The listing builds one solid part. Answer for the finished solid, in the listing's coordinates (mm). Face numbers are marked on the shaded views. Give positions to 0.01 mm unless a question says otherwise; leave off trailing zeros. Loops run counter-clockwise (first coordinate to the right, second up) from the corner with the lowest first, then second, coordinate; pieces in that order, holes last. Notation, with made-up numbers: M 31,52 L 51,52 A15 ccw 51,62 Z; hole C -23.75,27.25 d4. An arc over 180 degrees is marked long. Return JSON: item names as keys, results as strings.
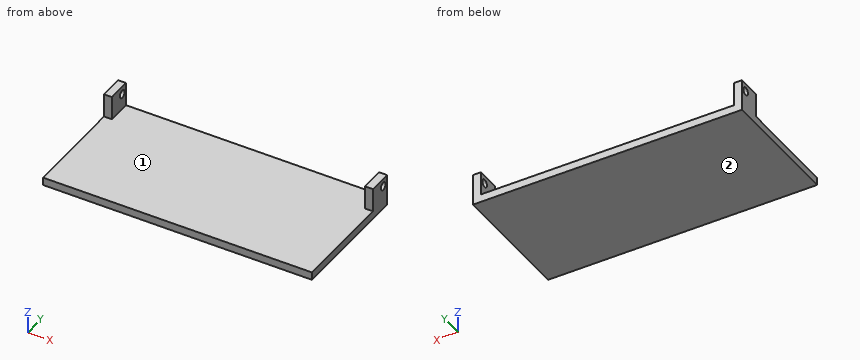
from build123d import *

# Parameters (mm, degrees)
SKETCH_1_W      = 170
SKETCH_1_H      = 80
EXTRUDE_1_DEPTH = 5
SKETCH_2_W      = 20
SKETCH_2_H      = 15
SKETCH_2_R      = 2.5
EXTRUDE_2_DEPTH = 5
EXTRUDE_START   = -5
SKETCH_3_W      = 20
SKETCH_3_H      = 15
SKETCH_3_R      = 2.5
EXTRUDE_3_DEPTH = 5


with BuildPart() as part:
    # 草图1 → 凸台-拉伸1 (new body)
    with BuildSketch(Plane.XY):
        with Locations((-2.943722944, -40)):
            Rectangle(SKETCH_1_W, SKETCH_1_H)
    extrude(amount=EXTRUDE_1_DEPTH)

    # 草图2 → 凸台-拉伸2 (add)
    with BuildSketch(Plane.ZY.offset(87.943722944)):
        with Locations((10, -7.5)):
            Rectangle(SKETCH_2_W, SKETCH_2_H)
        with Locations((15, -4)):
            Circle(SKETCH_2_R, mode=Mode.SUBTRACT)
    extrude(amount=-EXTRUDE_2_DEPTH)

    # 草图3 → 凸台-拉伸3 (add)
    with BuildSketch(Plane(origin=(82.056277056, 0, 0), x_dir=(0, 0, -1), z_dir=(1, 0, 0)).offset(EXTRUDE_START)):
        with Locations((-10, -7.5)):
            Rectangle(SKETCH_3_W, SKETCH_3_H)
        with Locations(Location((-15, -4, 0), (0, 0, 180))):
            Circle(SKETCH_3_R, mode=Mode.SUBTRACT)
    extrude(amount=EXTRUDE_3_DEPTH)


solid = part.part
(1) Straight lines are drawn through the part: line 1 along Y through (x, z) = (-84.1, 15); line 2 along Z through (x, y) = (28, -62); line 3 along X through (y, z) = (-10, 11.25). For each, find the intervals that lie inside material, in ascending order.
Values follow:
{"line 1": "-15 to -6.5, -1.5 to 0", "line 2": "0 to 5", "line 3": "-87.94 to -82.94, 77.06 to 82.06"}
(2) The part is cut by section C-C (x = -18.5). Determine the outline of the cut face in (y, z).
Values follow:
{"outline": "M -80,0 L 0,0 L 0,5 L -80,5 Z"}
(3) Given pin 1 (1.5 mm diameter, centred on x = -84, z = 15.5, fed in from -Y); pin 2 (3 mm diameter, centred on y = -4, z = 15, fed in from -X); pin 3 (4 mm diameter, centred on x = -55, y = -57.5, fed in from +Z), each flat-ended and moving along its own axis, determine where each tip first touches the part or whether it passes through.
Values follow:
{"pin 1": "y = -15", "pin 2": "through", "pin 3": "z = 5"}
(4) The part is cut by section B-B (z = 15). Determine the outline of the cut face in (x, y), and give its area (3 significant figures).
Values follow:
{"outline": "M -87.94,-15 L -82.94,-15 L -82.94,-6.5 L -87.94,-6.5 Z; M -87.94,-1.5 L -82.94,-1.5 L -82.94,0 L -87.94,0 Z; M 77.06,-15 L 82.06,-15 L 82.06,-6.5 L 77.06,-6.5 Z; M 77.06,-1.5 L 82.06,-1.5 L 82.06,0 L 77.06,0 Z", "area": "100 mm²"}
(5) The part is cut by section A-A (y = -4). Determine the outline of the cut face in (x, z), and give its area (3 significant figures).
Values follow:
{"outline": "M -87.94,0 L 82.06,0 L 82.06,12.5 L 77.06,12.5 L 77.06,5 L -82.94,5 L -82.94,12.5 L -87.94,12.5 Z; M -87.94,17.5 L -82.94,17.5 L -82.94,20 L -87.94,20 Z; M 77.06,17.5 L 82.06,17.5 L 82.06,20 L 77.06,20 Z", "area": "950 mm²"}
(6) Determine the mould class of the marked faces 1 and 2 for opening direction X: released by +X, released by -X, zero draft, split by the parting line, or undercut.
Values follow:
{"face 1": "undercut", "face 2": "zero draft"}
(7) The part is cut by section D-D (y = -64.5). Determine the outline of the cut face in (x, z), and give its area (3 significant figures).
Values follow:
{"outline": "M -87.94,0 L 82.06,0 L 82.06,5 L -87.94,5 Z", "area": "850 mm²"}
